Check sheet for the modelled part. Datum: model origin and axes. Units: mm. Face numbers are marked on the shaded views. Give positions to 0.01 mm unless a question says otherwise; leave off trailing zeros. Order: outer loops, then holes, each group sorted by start corner. A loop starts at its lowest first (then second) coordinate and runs counter-clockwise, first axis right, second up. Notation, with made-up numbers: (48, -28.75) - (78, -28.75) arc R6 ccw to (78, -23.75) - close; hole circle Ø2 at (52, 80.5). An arc over 180 degrees is marked (long way). Answer in a Markdown table with one row per item.
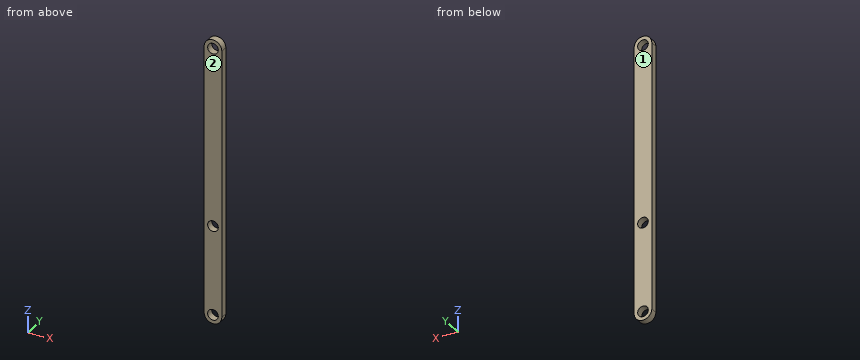
from build123d import *

# Parameters (mm, degrees)
F0_R     = 1.4986
F1_DEPTH = 1.0033


with BuildPart() as f1:
    # F0 (on Front) → F1 (new body, symmetric)
    with BuildSketch(Plane.XZ):
        with BuildLine():
            Line((2.4892, -37.5031), (2.4892, 37.5031))
            ThreePointArc((2.4892, 37.5031), (0, 39.9923), (-2.4892, 37.5031))
            Line((-2.4892, 37.5031), (-2.4892, -37.5031))
            ThreePointArc((-2.4892, -37.5031), (0, -39.9923), (2.4892, -37.5031))
        make_face()
        with Locations((0, -37.5031)):
            Circle(F0_R, mode=Mode.SUBTRACT)
        with Locations((0, -12.5095)):
            Circle(F0_R, mode=Mode.SUBTRACT)
        with Locations((0, 37.5031)):
            Circle(F0_R, mode=Mode.SUBTRACT)
    extrude(amount=F1_DEPTH, both=True)


solid = f1.part
(1) Cross-section at A-A, the plane x = 0. Record the cut outline in (y, z).
Geometry says:
| item | result |
|---|---|
| outline | (-1, -39.99) - (1, -39.99) - (1, -39) - (-1, -39) - close; (-1, -36) - (1, -36) - (1, -14.01) - (-1, -14.01) - close; (-1, -11.01) - (1, -11.01) - (1, 36) - (-1, 36) - close; (-1, 39) - (1, 39) - (1, 39.99) - (-1, 39.99) - close |
(2) Mould release check, pull along Y, two halves, no side actions. Record for the marked faces 1 and 2: pulls with the +Y half, pulls with the -Y half, needs draft (parallel to the pull), parting line crosses it, or undercut.
Geometry says:
| item | result |
|---|---|
| face 1 | pulls with the +Y half |
| face 2 | pulls with the -Y half |
(3) Thickness scan on L1, parallel to Z at x = 0, y = -0.45; L2, parallel to Z at x = 0.75, y = 0.7; L3, parallel to X at y = 0.35, z = -12. Record the ranges inside material, lowest first.
Geometry says:
| item | result |
|---|---|
| L1 | -39.99 to -39, -36 to -14.01, -11.01 to 36, 39 to 39.99 |
| L2 | -39.88 to -38.8, -36.21 to -13.81, -11.21 to 36.21, 38.8 to 39.88 |
| L3 | -2.49 to -1.41, 1.41 to 2.49 |
(4) Cross-section at B-B, the plane y = 0.2. Record the cut outline in (x, z).
Geometry says:
| item | result |
|---|---|
| outline | (-2.49, -37.5) arc R2.49 ccw to (2.49, -37.5) - (2.49, 37.5) arc R2.49 ccw to (-2.49, 37.5) - close; hole circle Ø3 at (0, -37.5); hole circle Ø3 at (0, -12.51); hole circle Ø3 at (0, 37.5) |
